Part model, mm, in its own coordinate system. Face numbers are marked on the shaded views. A direction names the side the tool comes from. Coordinates: 2 decimals unless noted, no trailing zeros. Loops run counter-clockwise (first coordinate to the right, second up) from the corner with the lowest first, then second, coordinate; pieces in that order, holes last. Notation, with made-up numbers: M 38,70 L 88,70 A13 cw 88,87 Z; hole C 34,-27.5 d9. An arc over 180 degrees is marked long. Use a Markdown table: item, result. Add a question column.
1) Band-saw the part on D-D (x = 8.75). List the corners of the cut face in (y, z).
2) Tool access for the marked faces 1 and 2: list every direction of +Z, -Z, +X, -X, +Y, -Y with a clear straight run to the whole face (end or side of a thin tool).
3) Band-saw the part on A-A (z = 11). List the corners of the cut face in (x, y) (3 decimals), plus the area to 3 significant figures.
4) Band-saw the part on C-C (y = -1.75). List the corners of the cut face in (x, z), plus the area to 3 significant figures.
5) Pull direction Y, two halves, no side cores. Call the marked faces 3, 4 and 5: released by +Y, released by -Y, zero draft, split by the parting line, or undercut.
6) Wall check: probe 1 along Y at (x, z) = (1.2, 11); probe 2 along Z at (x, y) = (2.4, -12.5); probe 3 along X at (y, z) = (-21, 10). Give the ranges that are in metal, low to high. Write a range as from..to.
7) Pin check, flat tips, straight feed: pin 1 Ø5.5 at (y, z) = (-12.5, 11) entering from +X; pin 2 Ø4 at (y, z) = (-11.5, 11.5) entering from -X; pin 3 Ø3.5 at (y, z) = (-24, 11) entering from +X; pin 4 Ø0.5 at (x, y) = (3.5, -12) entering from +Z. Stop position of each tip, or through.
8) Band-saw the part on B-B (y = -12.5). List the corners of the cut face in (x, z).
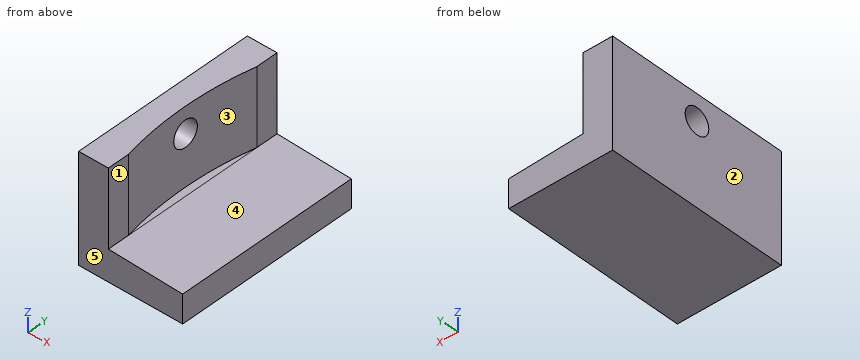
from build123d import *

# Parameters (mm, degrees)
F1_DEPTH = 25
F2_R     = 1.75
F3_DEPTH = 14.001
F5_DEPTH = 10.3


with BuildPart() as f1:
    # F0 (on Front) → F1 (new body)
    with BuildSketch(Plane.XZ):
        Polygon((0, 14.5), (0, 0), (14, 0), (14, 3.8), (4, 4.2), (4, 14.5), align=None)
    extrude(amount=F1_DEPTH)

    # F2 (on face) → F3 (cut, through all)
    with BuildSketch(Plane(origin=(0, 0, 0), x_dir=(0, -1, 0), z_dir=(-1, 0, 0))):
        with Locations((12.5, 11)):
            Circle(F2_R)
    extrude(amount=-F3_DEPTH, mode=Mode.SUBTRACT)

    # F4 (on face) → F5 (cut, through all)
    with BuildSketch(Plane.XY.offset(14.5)):
        with BuildLine():
            Line((4, -22), (4, -3))
            ThreePointArc((4, -3), (3, -12.5), (4, -22))
        make_face()
    extrude(amount=-F5_DEPTH, mode=Mode.SUBTRACT)


solid = f1.part
Entries:
| question | item | result |
|---|---|---|
| 1 | outline | M -25,0 L 0,0 L 0,4.01 L -25,4.01 Z |
| 2 | face 1 | +Z, +X, +Y, -Y |
| 2 | face 2 | +Z, -Z, -X, +Y, -Y |
| 3 | outline | M 0,-25 L 4,-25 L 4,-22 A45.625 cw 3.034,-14.25 L 0,-14.25 Z; M 0,-10.75 L 3.034,-10.75 A45.625 cw 4,-3 L 4,0 L 0,0 Z |
| 3 | area | 76.8 mm2 |
| 4 | outline | M 0,0 L 14,0 L 14,3.8 L 4,4.2 L 4,14.5 L 0,14.5 Z |
| 4 | area | 98.0 mm2 |
| 5 | face 3 | undercut |
| 5 | face 4 | zero draft |
| 5 | face 5 | released by -Y |
| 6 | probe 1 | -25..-14.25, -10.75..0 |
| 6 | probe 2 | 0..9.25, 12.75..14.5 |
| 6 | probe 3 | 0..3.8 |
| 7 | pin 1 | x = 3.08 |
| 7 | pin 2 | x = 0 |
| 7 | pin 3 | x = 4 |
| 7 | pin 4 | z = 4.2 |
| 8 | outline | M 0,0 L 14,0 L 14,3.8 L 4,4.2 L 3,4.2 L 3,9.25 L 0,9.25 Z; M 0,12.75 L 3,12.75 L 3,14.5 L 0,14.5 Z |
